from build123d import *

# Parameters (mm, degrees)
BOSS_EXTRUDE1_DEPTH         = 5.0292
SKETCH2_W                   = 34.036
SKETCH2_H                   = 8.89
BOSS_EXTRUDE2_DEPTH         = 32.9692
CUT_EXTRUDE1_DEPTH          = 61.762903104
CUT_EXTRUDE1_DEPTH_BACK     = 61.762903104
F_1_4_0_25_DIAMETER_HOLE1_D = 6.35
SKETCH7_R                   = 5.55625
CUT_EXTRUDE2_DEPTH          = 47.642102064
F_4_40_TAPPED_HOLE1_D       = 2.2606


with BuildPart() as part:
    # Sketch1 → Boss-Extrude1 (new body)
    with BuildSketch(Plane(origin=(0, 0, 0), x_dir=(1, 0, 0), z_dir=(0, 1, 0))):
        Polygon((-27.051, 7.874), (-17.018, 7.874), (-17.018, 16.860446287), (17.018, 16.860446287), (17.018, 7.874), (27.051, 7.874), (27.051, -7.874), (12.7, -16.159553713), (-12.7, -16.159553713), (-27.051, -7.874), align=None)
    extrude(amount=BOSS_EXTRUDE1_DEPTH)

    # Sketch2 → Boss-Extrude2 (add)
    with BuildSketch(Plane(origin=(0, 0, 0), x_dir=(1, 0, 0), z_dir=(0, 1, 0))):
        with Locations((0, 21.305446287)):
            Rectangle(SKETCH2_W, SKETCH2_H)
    extrude(amount=BOSS_EXTRUDE2_DEPTH)

    # Sketch3 → Cut-Extrude1 (cut, two sides: drawn at the far end of the back side and taken through both)
    with BuildSketch(Plane(origin=(17.018, 0, 0), x_dir=(0, 0, -1), z_dir=(1, 0, 0)).offset(-CUT_EXTRUDE1_DEPTH_BACK)):
        Polygon((66.671605927, 114.880744481), (25.750446287, 18.034), (18.130446287, 0), (-22.790713353, -96.846744481), (170.902775608, -178.68906376), (260.365094888, 33.038425201), align=None)
    extrude(amount=CUT_EXTRUDE1_DEPTH + CUT_EXTRUDE1_DEPTH_BACK, mode=Mode.SUBTRACT)

    # 1/4 (0.25) Diameter Hole1 (through all)
    with Locations(Plane.XY.offset(-16.860446287)):
        with Locations((-10.16, 27.178), (10.16, 27.178)):
            Hole(F_1_4_0_25_DIAMETER_HOLE1_D / 2)

    # Sketch7 → Cut-Extrude2 (cut, through all)
    with BuildSketch(Plane(origin=(0, 5.0292, 0), x_dir=(1, 0, 0), z_dir=(0, 1, 0))):
        with Locations(Location((0, -4.064, 0), (0, 0, 270))):
            Circle(SKETCH7_R)
    extrude(amount=-CUT_EXTRUDE2_DEPTH, mode=Mode.SUBTRACT)

    # #4-40 Tapped Hole1 (through all)
    with Locations(Plane(origin=(0, 5.0292, 0), x_dir=(1, 0, 0), z_dir=(0, 1, 0))):
        with Locations((0, 0), (-22.5, -4.064), (22.5, -4.064)):
            Hole(F_4_40_TAPPED_HOLE1_D / 2)


solid = part.part
Model file for the job. Use its own axes, mm. A direction names the side the tool comes from. Give positions to 0.01 mm unless a question says otherwise; leave off trailing zeros. Loops run counter-clockwise (first coordinate to the right, second up) from the corner with the lowest first, then second, coordinate; pieces in that order, holes last.
1) Saw through at C-C (y = 4). Write the cut outline in (x, z), plus the area to 3 significant figures.
2) Flat gauge pins, fed straight in: pin 1 Ø4 at (x, y) = (-23, 3) entering from -Z; pin 2 Ø9 at (y, z) = (24, -18.5) entering from +X; pin 3 Ø10 at (x, y) = (-10.16, 27.178) entering from -Z; pin 4 Ø1.5 at (x, z) = (-7, 8.5) entering from +Y. Where does each tip first touch, or does it go through?
3) Saw through at D-D (y = 26). Write the cut outline in (x, z).
4) Pull direction Z, two halves, no side cores. Call faces 5 (the flat face through (17.018, 16, -21)), 6 (the cylindrical face through (4.685, 2.55, 7.051)), 7 (the flat face through (-0.238, 9.143, -21.994)): +Z half, -Z half, draft (parallel to the pull), parting line (faces both ways), or undercut.
5) Saw through at B-B (z = 1). Write the cut outline in (x, y).
6) Tool access for faces 1 (the flat face through (0, 19, -16.86)), 2 (the flat face through (22, 2, -7.874)), 3 (the cylindrical face through (8.695, 24.361, -21.368)), 4 (the flat face through (-17.018, 16, -21)): list every direction of +Z, -Z, +X, -X, +Y, -Y with a clear straight run to the whole face (end or side of a thin tool).
7) Wall check: line 1 (Y direction, x = -17.5, z = -6); line 2 (Z direction, x = -0.5, y = 18); line 3 (X direction, y = 4.5, z = -15). Give the ranges that are in metal, low to high.
8) Saw through at A-A (x = 0). Write the cut outline in (y, z).
Answer block:
1. outline: (-27.05, -7.87) - (-17.02, -7.87) - (-17.02, -19.82) - (17.02, -19.82) - (17.02, -7.87) - (27.05, -7.87) - (27.05, 7.87) - (12.7, 16.16) - (-12.7, 16.16) - (-27.05, 7.87) - close; hole circle Ø2.26 at (-22.5, 4.06); hole circle Ø11.11 at (0, 4.06); hole circle Ø2.26 at (22.5, 4.06)
1. area: 1,480 mm2
2. pin 1: stops at z = -7.87
2. pin 2: stops at x = 17.02
2. pin 3: stops at z = -25.75
2. pin 4: stops at y = 5.03
3. outline: (-17.02, -25.75) - (-13.11, -25.75) - (-13.11, -16.86) - (-17.02, -16.86) - close; (-7.21, -25.75) - (7.21, -25.75) - (7.21, -16.86) - (-7.21, -16.86) - close; (13.11, -25.75) - (17.02, -25.75) - (17.02, -16.86) - (13.11, -16.86) - close
4. face 5: draft
4. face 6: undercut
4. face 7: -Z half
5. outline: (-27.05, 0) - (-4.64, 0) - (-4.64, 5.03) - (-27.05, 5.03) - close; (4.64, 0) - (27.05, 0) - (27.05, 5.03) - (4.64, 5.03) - close
6. face 1: +Z, +X, -X, +Y
6. face 2: -Z, +X, +Y, -Y
6. face 3: +Z, -Z
6. face 4: -Z, -X, +Y, -Y
7. line 1: y = 0 to 5.03
7. line 2: z = -25.74 to -16.86
7. line 3: x = -17.02 to 17.02
8. outline: (0, -18.13) - (18.03, -25.75) - (32.97, -25.75) - (32.97, -16.86) - (5.03, -16.86) - (5.03, -1.49) - (0, -1.49) - close; (0, 9.62) - (5.03, 9.62) - (5.03, 16.16) - (0, 16.16) - close
